```python
from build123d import *

# Parameters (mm, degrees)
SKETCH_1_R      = 2.5
EXTRUDE_1_DEPTH = 650


with BuildPart() as part:
    # 草图1 → 凸台-拉伸1 (new body)
    with BuildSketch(Plane(origin=(0, 0, 0), x_dir=(1, 0, 0), z_dir=(0, 1, 0))):
        with BuildLine():
            Line((-3.6, 10), (-8.5, 10))
            ThreePointArc((-8.5, 10), (-9.560660172, 9.560660172), (-10, 8.5))
            Line((-10, 8.5), (-10, 3.6))
            Line((-10, 3.6), (-9.4, 3.6))
            Line((-9.4, 3.6), (-9.4, 3.1))
            Line((-9.4, 3.1), (-8.2, 3.1))
            Line((-8.2, 3.1), (-8.2, 5.5))
            Line((-8.2, 5.5), (-6.348528137, 5.5))
            Line((-6.348528137, 5.5), (-3.5, 2.651471863))
            Line((-3.5, 2.651471863), (-3.5, -2.651471863))
            Line((-3.5, -2.651471863), (-6.348528137, -5.5))
            Line((-6.348528137, -5.5), (-8.2, -5.5))
            Line((-8.2, -5.5), (-8.2, -3.1))
            Line((-8.2, -3.1), (-9.4, -3.1))
            Line((-9.4, -3.1), (-9.4, -3.6))
            Line((-9.4, -3.6), (-10, -3.6))
            Line((-10, -3.6), (-10, -8.5))
            ThreePointArc((-10, -8.5), (-9.560660172, -9.560660172), (-8.5, -10))
            Line((-8.5, -10), (-3.6, -10))
            Line((-3.6, -10), (-3.6, -9.4))
            Line((-3.6, -9.4), (-3.1, -9.4))
            Line((-3.1, -9.4), (-3.1, -8.2))
            Line((-3.1, -8.2), (-5.5, -8.2))
            Line((-5.5, -8.2), (-5.5, -6.348528137))
            Line((-5.5, -6.348528137), (-2.651471863, -3.5))
            Line((-2.651471863, -3.5), (2.651471863, -3.5))
            Line((2.651471863, -3.5), (5.5, -6.348528137))
            Line((5.5, -6.348528137), (5.5, -8.2))
            Line((5.5, -8.2), (3.1, -8.2))
            Line((3.1, -8.2), (3.1, -9.4))
            Line((3.1, -9.4), (3.6, -9.4))
            Line((3.6, -9.4), (3.6, -10))
            Line((3.6, -10), (8.5, -10))
            ThreePointArc((8.5, -10), (9.560660172, -9.560660172), (10, -8.5))
            Line((10, -8.5), (10, -3.6))
            Line((10, -3.6), (9.4, -3.6))
            Line((9.4, -3.6), (9.4, -3.1))
            Line((9.4, -3.1), (8.2, -3.1))
            Line((8.2, -3.1), (8.2, -5.5))
            Line((8.2, -5.5), (6.348528137, -5.5))
            Line((6.348528137, -5.5), (3.5, -2.651471863))
            Line((3.5, -2.651471863), (3.5, 2.651471863))
            Line((3.5, 2.651471863), (6.348528137, 5.5))
            Line((6.348528137, 5.5), (8.2, 5.5))
            Line((8.2, 5.5), (8.2, 3.1))
            Line((8.2, 3.1), (9.4, 3.1))
            Line((9.4, 3.1), (9.4, 3.6))
            Line((9.4, 3.6), (10, 3.6))
            Line((10, 3.6), (10, 8.5))
            ThreePointArc((10, 8.5), (9.560660172, 9.560660172), (8.5, 10))
            Line((8.5, 10), (3.6, 10))
            Line((3.6, 10), (3.6, 9.4))
            Line((3.6, 9.4), (3.1, 9.4))
            Line((3.1, 9.4), (3.1, 8.2))
            Line((3.1, 8.2), (5.5, 8.2))
            Line((5.5, 8.2), (5.5, 6.348528137))
            Line((5.5, 6.348528137), (2.651471863, 3.5))
            Line((2.651471863, 3.5), (-2.651471863, 3.5))
            Line((-2.651471863, 3.5), (-5.5, 6.348528137))
            Line((-5.5, 6.348528137), (-5.5, 8.2))
            Line((-5.5, 8.2), (-3.1, 8.2))
            Line((-3.1, 8.2), (-3.1, 9.4))
            Line((-3.1, 9.4), (-3.6, 9.4))
            Line((-3.6, 9.4), (-3.6, 10))
        make_face()
        with Locations(Location((0, 0, 0), (0, 0, 270))):
            Circle(SKETCH_1_R, mode=Mode.SUBTRACT)
        with BuildLine():
            Line((-7.4, 9.1), (-8.1, 9.1))
            ThreePointArc((-8.1, 9.1), (-8.807106781, 8.807106781), (-9.1, 8.1))
            Line((-9.1, 8.1), (-9.1, 7.4))
            ThreePointArc((-9.1, 7.4), (-8.807106781, 6.692893219), (-8.1, 6.4))
            Line((-8.1, 6.4), (-7.4, 6.4))
            ThreePointArc((-7.4, 6.4), (-6.692893219, 6.692893219), (-6.4, 7.4))
            Line((-6.4, 7.4), (-6.4, 8.1))
            ThreePointArc((-6.4, 8.1), (-6.692893219, 8.807106781), (-7.4, 9.1))
        make_face(mode=Mode.SUBTRACT)
        with BuildLine():
            Line((9.1, 7.4), (9.1, 8.1))
            ThreePointArc((9.1, 8.1), (8.807106781, 8.807106781), (8.1, 9.1))
            Line((8.1, 9.1), (7.4, 9.1))
            ThreePointArc((7.4, 9.1), (6.692893219, 8.807106781), (6.4, 8.1))
            Line((6.4, 8.1), (6.4, 7.4))
            ThreePointArc((6.4, 7.4), (6.692893219, 6.692893219), (7.4, 6.4))
            Line((7.4, 6.4), (8.1, 6.4))
            ThreePointArc((8.1, 6.4), (8.807106781, 6.692893219), (9.1, 7.4))
        make_face(mode=Mode.SUBTRACT)
        with BuildLine():
            Line((7.4, -9.1), (8.1, -9.1))
            ThreePointArc((8.1, -9.1), (8.807106781, -8.807106781), (9.1, -8.1))
            Line((9.1, -8.1), (9.1, -7.4))
            ThreePointArc((9.1, -7.4), (8.807106781, -6.692893219), (8.1, -6.4))
            Line((8.1, -6.4), (7.4, -6.4))
            ThreePointArc((7.4, -6.4), (6.692893219, -6.692893219), (6.4, -7.4))
            Line((6.4, -7.4), (6.4, -8.1))
            ThreePointArc((6.4, -8.1), (6.692893219, -8.807106781), (7.4, -9.1))
        make_face(mode=Mode.SUBTRACT)
        with BuildLine():
            Line((-9.1, -7.4), (-9.1, -8.1))
            ThreePointArc((-9.1, -8.1), (-8.807106781, -8.807106781), (-8.1, -9.1))
            Line((-8.1, -9.1), (-7.4, -9.1))
            ThreePointArc((-7.4, -9.1), (-6.692893219, -8.807106781), (-6.4, -8.1))
            Line((-6.4, -8.1), (-6.4, -7.4))
            ThreePointArc((-6.4, -7.4), (-6.692893219, -6.692893219), (-7.4, -6.4))
            Line((-7.4, -6.4), (-8.1, -6.4))
            ThreePointArc((-8.1, -6.4), (-8.807106781, -6.692893219), (-9.1, -7.4))
        make_face(mode=Mode.SUBTRACT)
    extrude(amount=EXTRUDE_1_DEPTH)


solid = part.part
```
For this review, take the finished solid that the model builds, in its own axes (mm). Give positions to 0.01 mm unless a question says otherwise; leave off trailing zeros.
Item 1: Wall thickness on probe 1 along X at (y, z) = (545, -7); probe 2 along X at (y, z) = (467.5, -8): over which ranges is each line inside the solid? List them lowest first.
Item 2: Take a section at A-A (y = 357). Give the number of separate pieces and of enclosed holes in the cut face, and give its area (3 significant figures).
Item 3: Insertion check: P1, Ø0.7, axis at y = 252.5, z = -9.5, coming from the -X side; P2, Ø0.5, axis at y = 366, z = 9.5, coming from the +X side; P3, Ø3, axis at y = 144.5, z = -1.5, coming from the +X side; P4, Ø1, axis at x = -1.5, z = -4.5, coming from the +Y side. Each pin has a flat end and moves straight along its axis. Give the tip position at first contact, or say it passes through.
Established:
1. probe 1: x = -10 to -9.02, -6.48 to -5.5, 5.5 to 6.48, 9.02 to 10
1. probe 2: x = -10 to -9.1, -6.4 to -5.5, 5.5 to 6.4, 9.1 to 10
2. separate pieces: 1
2. enclosed holes: 5
2. area: 131 mm2
3. P1: stops at x = -9.85
3. P2: stops at x = 9.8
3. P3: stops at x = 3.85
3. P4: passes through
